CAD build for the part. Positions are in the model's coordinates, mm. Face numbers are marked on the shaded views. A direction names the side the tool comes from. Round coordinates to 2 decimals unless told otherwise and drop trailing zeros. Order: outer loops, then holes, each group sorted by start corner. A loop starts at its lowest first (then second) coordinate and runs counter-clockwise, first axis right, second up. Notation, with made-up numbers: M 1,-23 L 9,-23 A9 cw 9,-10 Z; hole C 16.5,87 d9. An arc over 180 degrees is marked long. Answer as CSV lines item,"result". Start each with the question number.
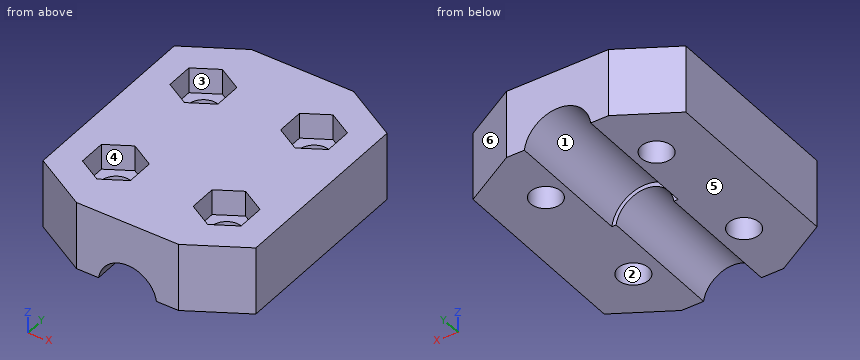
```python
from build123d import *

# Parameters (mm, degrees)
SCHIZZO1_R         = 1.8
MAIN_BODY_DEPTH    = 8
SCHIZZO2_R         = 3.925
THREADED_ROD_DEPTH = 15
SCHIZZO4_R         = 3.4325
MOTOR_SHAFT_DEPTH  = 15
NUT_RECESS_DEPTH   = 3


with BuildPart() as part:
    # Schizzo1 → Main Body (new body)
    with BuildSketch(Plane.XY):
        Polygon((12.5, -11.24722325), (12.5, 11.24722325), (6, 15), (-6, 15), (-12.5, 11.24722325), (-12.5, -11.24722325), (-6, -15), (6, -15), align=None)
        with Locations((-6.5, 7.5)):
            Circle(SCHIZZO1_R, mode=Mode.SUBTRACT)
        with Locations((6.5, -7.5)):
            Circle(SCHIZZO1_R, mode=Mode.SUBTRACT)
        with Locations(Location((-6.5, -7.5, 0), (0, 0, 180))):
            Circle(SCHIZZO1_R, mode=Mode.SUBTRACT)
        with Locations(Location((6.5, 7.5, 0), (0, 0, 180))):
            Circle(SCHIZZO1_R, mode=Mode.SUBTRACT)
    extrude(amount=MAIN_BODY_DEPTH)

    # Schizzo2 → Threaded rod (cut)
    with BuildSketch(Plane(origin=(0, 15, 0), x_dir=(1, 0, 0), z_dir=(0, 1, 0))):
        with Locations((0, 0.5)):
            Circle(SCHIZZO2_R)
    extrude(amount=-THREADED_ROD_DEPTH, mode=Mode.SUBTRACT)

    # Schizzo4 → Motor shaft (cut)
    with BuildSketch(Plane.XZ.offset(15)):
        with Locations((0, -0.5)):
            Circle(SCHIZZO4_R)
    extrude(amount=-MOTOR_SHAFT_DEPTH, mode=Mode.SUBTRACT)

    # Schizzo5 → Nut recess (cut)
    with BuildSketch(Plane.XY.offset(8)):
        Polygon((-9.314582562, -5.875), (-6.5, -4.25), (-3.685417438, -5.875), (-3.685417438, -9.125), (-6.5, -10.75), (-9.314582562, -9.125), align=None)
        Polygon((6.5, -4.25), (3.685417438, -5.875), (3.685417438, -9.125), (6.5, -10.75), (9.314582562, -9.125), (9.314582562, -5.875), align=None)
        Polygon((-6.5, 4.25), (-3.685417438, 5.875), (-3.685417438, 9.125), (-6.5, 10.75), (-9.314582562, 9.125), (-9.314582562, 5.875), align=None)
        Polygon((9.314582562, 5.875), (6.5, 4.25), (3.685417438, 5.875), (3.685417438, 9.125), (6.5, 10.75), (9.314582562, 9.125), align=None)
    extrude(amount=-NUT_RECESS_DEPTH, mode=Mode.SUBTRACT)


solid = part.part
```
Q1. Probe line 1 along Y through (x, z) = (-6.5, 1.2); line 2 along Y through (x, z) = (-9.25, 6.25); line 3 along X through (y, z) = (-6.75, 2). List the from-to ranges inside material, lowest first. Write a range as from..to.
Q2. Drop a flat-ended pin along its axis: P1, Ø1.7, axis at x = 5.5, y = 7.5, coming from the +Z side. Give the stop position or say it passes through.
Q3. Mould opens along Y. For the marked faces 4, 5 and 6 say: +Y half, -Y half, draft (parallel to the pull), parting line (faces both ways), or undercut.
Q4. Band-saw the part on A-A, the plane y = -7.5. Write the cut outline in (x, z) (1 decimal).
Q5. Band-saw the part on B-B, the plane z = 4. Write the cut outline in (x, y).
Q6. Band-saw the part on D-D, the plane x = 0. Write the cut outline in (y, z) (1 decimal), then the cut area to 3 significant figures.
Q7. Tool access for the marked faces 1, 2 and 3: list every direction of +Z, -Z, +X, -X, +Y, -Y with a clear straight run to the whole face (end or side of a thin tool).
Q8. Band-saw the part on C-C, the plane y = 7.5. Write the cut outline in (x, z) (3 decimals), then the cut area to 3 significant figures.
Answer:
1,line 1,"y = -14.71..-9.3, -5.7..5.7, 9.3..14.71"
1,line 2,"y = -13.12..-9.16, -5.84..5.84, 9.16..13.12"
1,line 3,"x = -12.5..-8.14, -4.86..-2.35, 2.35..4.86, 8.14..12.5"
2,P1,"stops at z = 5"
3,face 4,"undercut"
3,face 5,"draft"
3,face 6,"+Y half"
4,outline,"M -12.5,0 L -8.3,0 L -8.3,5 L -9.3,5 L -9.3,8 L -12.5,8 Z; M -4.7,0 L -3.4,0 A3.4 cw 3.4,0 L 4.7,0 L 4.7,5 L 3.7,5 L 3.7,8 L -3.7,8 L -3.7,5 L -4.7,5 Z; M 8.3,0 L 12.5,0 L 12.5,8 L 9.3,8 L 9.3,5 L 8.3,5 Z"
5,outline,"M -12.5,-11.25 L -6,-15 L 6,-15 L 12.5,-11.25 L 12.5,11.25 L 6,15 L -6,15 L -12.5,11.25 Z; hole C -6.5,-7.5 d3.6; hole C -6.5,7.5 d3.6; hole C 6.5,-7.5 d3.6; hole C 6.5,7.5 d3.6"
6,outline,"M -15,2.9 L 0,2.9 L 0,3.4 L 15,3.4 L 15,8 L -15,8 Z"
6,area,"145 mm^2"
7,face 1,"-Z, +Y"
7,face 2,"+Z, -Z"
7,face 3,"+Z"
8,outline,"M -12.5,0 L -8.3,0 L -8.3,5 L -9.315,5 L -9.315,8 L -12.5,8 Z; M -4.7,0 L -3.893,0 A3.925 cw 3.893,0 L 4.7,0 L 4.7,5 L 3.685,5 L 3.685,8 L -3.685,8 L -3.685,5 L -4.7,5 Z; M 8.3,0 L 12.5,0 L 12.5,8 L 9.315,8 L 9.315,5 L 8.3,5 Z"
8,area,"110 mm^2"
